from build123d import *

# Parameters (mm, degrees)
SKETCH1_R                                      = 38.1
SKETCH1_R_2                                    = 20
BOSS_EXTRUDE1_DEPTH                            = 75
BOSS_EXTRUDE2_START                            = -8
SKETCH2_R                                      = 38.1
SKETCH2_R_2                                    = 20
BOSS_EXTRUDE2_DEPTH                            = 8
CSK_FOR_8_FLAT_HEAD_MACHINE_SCREW2_D           = 4.4958
CSK_FOR_8_FLAT_HEAD_MACHINE_SCREW2_CSINK_D     = 10.1713792
CSK_FOR_8_FLAT_HEAD_MACHINE_SCREW2_CSINK_ANGLE = 82
BOSS_EXTRUDE3_START                            = -63
SKETCH5_R                                      = 20
SKETCH5_R_2                                    = 16
BOSS_EXTRUDE3_DEPTH                            = 51
TAP_DRILL_FOR_M5X0_8_TAP1_D                    = 4.2


with BuildPart() as part:
    # Sketch1 → Boss-Extrude1 (new body)
    with BuildSketch(Plane(origin=(0, 0, 0), x_dir=(1, 0, 0), z_dir=(0, 1, 0))):
        with Locations(Location((0, 0, 0), (0, 0, 270))):
            Circle(SKETCH1_R)
        with Locations(Location((0, 0, 0), (0, 0, 270))):
            Circle(SKETCH1_R_2, mode=Mode.SUBTRACT)
    extrude(amount=BOSS_EXTRUDE1_DEPTH)

    # Sketch2 → Boss-Extrude2 (add)
    # profile 1 of 2: a face of its own
    with BuildSketch(Plane(origin=(0, 75, 0), x_dir=(1, 0, 0), z_dir=(0, 1, 0)).offset(BOSS_EXTRUDE2_START)):
        with BuildLine():
            ThreePointArc((57.15, 0), (-20.392382431, 53.387950315), (-42.597094971, -38.1))
            Line((-42.597094971, -38.1), (0, -38.1))
            Line((0, -38.1), (42.597094971, -38.1))
            ThreePointArc((42.597094971, -38.1), (53.387950315, -20.392382431), (57.15, 0))
        make_face()
        with BuildLine():
            ThreePointArc((38.1, 0), (26.940768363, -26.940768363), (0, -38.1))
            ThreePointArc((0, -38.1), (-26.940768363, 26.940768363), (38.1, 0))
        make_face(mode=Mode.SUBTRACT)
    # profile 2 of 2: a face of its own
    with BuildSketch(Plane(origin=(0, 75, 0), x_dir=(1, 0, 0), z_dir=(0, 1, 0)).offset(BOSS_EXTRUDE2_START)):
        with Locations(Location((0, 0, 0), (0, 0, 270))):
            Circle(SKETCH2_R)
        with Locations(Location((0, 0, 0), (0, 0, 270))):
            Circle(SKETCH2_R_2, mode=Mode.SUBTRACT)
    extrude(amount=BOSS_EXTRUDE2_DEPTH)

    # CSK for #8 Flat Head Machine Screw2 (through all)
    with Locations(Plane(origin=(0, 75, 0), x_dir=(1, 0, 0), z_dir=(0, 1, 0))):
        with Locations((-41.244459855, -23.8125), (-41.244459855, 23.8125), (0, 47.625), (41.244459855, 23.8125), (41.244459855, -23.8125), (0, -47.625)):
            CounterSinkHole(CSK_FOR_8_FLAT_HEAD_MACHINE_SCREW2_D / 2, CSK_FOR_8_FLAT_HEAD_MACHINE_SCREW2_CSINK_D / 2, counter_sink_angle=CSK_FOR_8_FLAT_HEAD_MACHINE_SCREW2_CSINK_ANGLE)

    # Sketch5 → Boss-Extrude3 (add)
    with BuildSketch(Plane(origin=(0, 75, 0), x_dir=(1, 0, 0), z_dir=(0, 1, 0)).offset(BOSS_EXTRUDE3_START)):
        with Locations(Location((0, 0, 0), (0, 0, 270))):
            Circle(SKETCH5_R)
        with Locations(Location((0, 0, 0), (0, 0, 270))):
            Circle(SKETCH5_R_2, mode=Mode.SUBTRACT)
    extrude(amount=BOSS_EXTRUDE3_DEPTH)

    # Tap Drill for M5x0.8 Tap1 (through all)
    with Locations(Plane(origin=(0, 75, 0), x_dir=(1, 0, 0), z_dir=(0, 1, 0))):
        with Locations((0, 23.5), (0, -23.5)):
            Hole(TAP_DRILL_FOR_M5X0_8_TAP1_D / 2)


solid = part.part
Model file for the job. Use its own axes, mm. A direction names the side the tool comes from. Round coordinates to 2 decimals unless told otherwise and drop trailing zeros. Loops run counter-clockwise (first coordinate to the right, second up) from the corner with the lowest first, then second, coordinate; pieces in that order, holes last. Notation, with made-up numbers: (-18, 65.25) -> (2, 65.25) arc R23 cw to (2, 94.25) -> close; hole circle Ø2 at (-2, 9.5). An arc over 180 degrees is marked (long way). Answer as CSV lines item,"result". Start each with the question number.
1) Mould opens along Z. For faces 4 (the face through (-23.183, 33.031, -30.235)), 5 (the face through (-1, 71, 38.1)), 6 (the face through (-1, 75, -21)), 7 (the face through (-19.524, 68.916, -4.336)) say: +Z half, -Z half, draft (parallel to the pull), parting line (faces both ways), or undercut.
2) Pin check, flat tips, straight feed: P1, Ø7, axis at x = 41.24, z = -23.81, coming from the -Y side; P2, Ø7, axis at x = 41.24, z = 23.81, coming from the +Y side; P3, Ø6, axis at x = 14, y = 18, coming from the +Z side; P4, Ø5, axis at x = -16, z = 10, coming from the -Y side. Stop position of each tip, or through.
3) Probe line 1 along X through (y, z) = (70, -0.5); line 2 along X through (y, z) = (35.5, 1); line 3 along Y through (x, z) = (40, 17.5). List the from-to ranges inside material, lowest first.
4) Slice it at B-B (y = 50). List the corners of the cut face in (x, z), plus the area to 3 significant figures.
5) Tool access for faces 1 (the face through (-1, 67, -42)), 2 (the face through (42.901, 69.335, -25.332)), 3 (the face through (13.43, 63, -8.98)): list every direction of +Z, -Z, +X, -X, +Y, -Y with a clear straight run to the whole face (end or side of a thin tool).
6) Slice it at D-D (x = -28). List the corners of the cut face in (y, z), plus the area to 3 significant figures.
7) Slice it at A-A (x = 12). List the corners of the cut face in (y, z), plus the area to 3 significant figures.
8) Slice it at C-C (z = -35). List the corners of the cut face in (x, y), plus the area to 3 significant figures.
Filled in:
1,face 4,"parting line"
1,face 5,"+Z half"
1,face 6,"draft"
1,face 7,"undercut"
2,P1,"stops at y = 67"
2,P2,"stops at y = 73.18"
2,P3,"stops at z = 36.48"
2,P4,"stops at y = 0"
3,line 1,"x = -57.15 to -19.99, 19.99 to 57.15"
3,line 2,"x = -38.09 to -15.97, 15.97 to 38.09"
3,line 3,"y = 67 to 75"
4,outline,"circle Ø76.2 at (0, 0); hole circle Ø32 at (0, 0); hole circle Ø4.2 at (0, -23.5); hole circle Ø4.2 at (0, 23.5)"
4,area,"3,730 mm2"
5,face 1,"-Y"
5,face 2,"+Y, -Y"
5,face 3,"+Y"
6,outline,"(0, -25.84) -> (67, -25.84) -> (67, -49.82) -> (75, -49.82) -> (75, 38.1) -> (67, 38.1) -> (67, 25.84) -> (0, 25.84) -> close"
6,area,"4,170 mm2"
7,outline,"(0, -36.16) -> (67, -36.16) -> (67, -55.88) -> (75, -55.88) -> (75, -16) -> (63, -16) -> (63, -10.58) -> (12, -10.58) -> (12, -16) -> (0, -16) -> close; (0, 16) -> (12, 16) -> (12, 10.58) -> (63, 10.58) -> (63, 16) -> (75, 16) -> (75, 38.1) -> (67, 38.1) -> (67, 36.16) -> (0, 36.16) -> close"
7,area,"3,750 mm2"
8,outline,"(-45.18, 67) -> (-15.05, 67) -> (-15.05, 0) -> (15.05, 0) -> (15.05, 67) -> (45.18, 67) -> (45.18, 75) -> (-45.18, 75) -> close"
8,area,"2,740 mm2"
